Can you work these out from the model? Positions are in its coordinate system, mm. A direction names the side the tool comes from. Coordinates: 2 decimals unless noted, no trailing zeros. Loops run counter-clockwise (first coordinate to the right, second up) from the corner with the lowest first, then second, coordinate; pieces in that order, holes last.
Autodesk Inventor part; units mm, degrees
ref_plane "YZ Plane" through (0, 0, 0) normal (1, 0, 0) x (0, 1, 0)
ref_plane "XZ Plane" through (0, 0, 0) normal (0, 1, 0) x (-1, 0, 0)
ref_plane "XY Plane" through (0, 0, 0) normal (0, 0, 1) x (1, 0, 0)
sketch "Sketch1" plane through (0, 0, 0) normal (0, 0, 1) x (1, 0, 0)
  line L0 (0, 0) -> (18.64, 0)
  line L1 (18.64, 0) -> (18.64, -7)
  line L2 (18.64, -7) -> (0, -7)
  line L3 (0, -7) -> (0, 0)
  circle A0 centre (3.95, -5.19) radius 1.75
  line L4 (9.32, 0) -> (9.32, 1.7268)
  line L5 (9.32, 0) -> (8.32, 0)
  line L6 (8.32, 0) -> (8.32, -6.4)
  line L7 (8.32, -6.4) -> (9.32, -6.4)
  line L8 (9.32, -6.4) -> (9.32, 0)
  circle A1 centre (14.69, -5.19) radius 1.75
  line L9 (10.32, 0) -> (10.32, -6.4)
  line L10 (10.32, -6.4) -> (9.32, -6.4)
  point P0 (8.82, -6.4)
  dimension "d0" = 18.64
  dimension "d1" = 7
  dimension "d2" = 5.19
  dimension "d3" = 3.5
  dimension "d4" = 3.95
  dimension "d5" = 0.6
  dimension "d6" = 1
extrude "Extrusion1" add sketch "Sketch1" along normal blind 1 contours L0 L6 L7 L10 L9 L1 L2 L3
sketch "Sketch2" plane through (0, 0, 1) normal (0, 0, 1) x (1, 0, 0)
  line L0 (0, -7) -> (18.64, -7)
  line L1 (18.64, -7) -> (18.64, 0)
  line L2 (18.64, 0) -> (10.32, 0)
  line L3 (10.32, -6.4) -> (8.32, -6.4)
  line L4 (8.32, -6.4) -> (8.32, 0)
  line L5 (8.32, 0) -> (0, 0)
  line L6 (0, 0) -> (0, -7)
  circle A0 centre (3.95, -5.19) radius 1.75
  circle A1 centre (14.69, -5.19) radius 1.75
  line L7 (8.32, 0) -> (0, 0)
  line L8 (8.32, -6.4) -> (8.32, 0)
  line L9 (0, 0) -> (8.32, 0)
  line L10 (8.32, 0) -> (8.32, -2.5)
  line L11 (8.32, -2.5) -> (0, -2.5)
  line L12 (0, -2.5) -> (0, 0)
  line L13 (9.32, 0) -> (9.32, -6.4)
  line L14 (18.64, -7) -> (18.64, 0)
  line L15 (9.32, 0) -> (18.64, 0)
  line L16 (18.64, 0) -> (18.64, -2.5)
  line L17 (18.64, -2.5) -> (9.32, -2.5)
  line L18 (9.32, -2.5) -> (9.32, 0)
  line L19 (10.32, 0) -> (10.32, -6.4)
  point P0 (0, -2.5)
  point P1 (10.32, -2.5)
  dimension "d9" = 2.5
  dimension "d10" = 2.5
extrude "Extrusion2" add sketch "Sketch2" along normal blind 18 contours L6 L5 L4 L11 | L17 L19 L2 L1
sketch "Sketch3" plane through (8.32, -6.4, 0) normal (1, 0, 0) x (0, 0, -1)
  line L0 (0, 0) -> (0, 6.4)
  line L1 (0, 6.4) -> (-19, 6.4)
  line L2 (-19, 3.9) -> (-19, 6.4)
  line L3 (-1, 3.9) -> (-19, 3.9)
  line L4 (-1, 0) -> (-1, 3.9)
  line L5 (0, 0) -> (-1, 0)
  line L6 (-1, 3.9) -> (-19, 3.9)
  line L7 (-19, 6.4) -> (-9, 6.4)
  line L8 (-9, 6.4) -> (-9, 3.9)
  line L9 (-9, 3.9) -> (-19, 3.9)
  line L10 (-19, 3.9) -> (-19, 6.4)
  point P0 (0, 6.4)
  dimension "d13" = 10
extrude "Extrusion3" add sketch "Sketch3" along normal blind 2 contours L8 L3 L2 L1
sketch "Sketch4" plane through (0, 0, 19) normal (0, 0, 1) x (1, 0, 0)
  line L0 (18.64, 0) -> (10.32, 0)
  line L1 (18.64, 0) -> (0, 0)
  line L2 (0, 0) -> (0, 100)
  line L3 (0, 100) -> (18.64, 100)
  line L4 (18.64, 100) -> (18.64, 0)
  line L5 (10.32, -2.5) -> (10.32, 0)
  line L6 (18.64, 0) -> (0, 0)
  line L7 (0, 0) -> (0, -2.5)
  line L8 (0, -2.5) -> (18.64, -2.5)
  line L9 (18.64, -2.5) -> (18.64, 0)
  dimension "d16" = 100
extrude "Extrusion4" add sketch "Sketch4" along normal blind 2
sketch "Sketch5" plane through (0, 0, 21) normal (0, 0, 1) x (1, 0, 0)
  circle A0 centre (12.82, 93) radius 1.5
  circle A1 centre (5.82, 93) radius 1.5
  line L0 (12.82, 93) -> (5.82, 93)
  line L1 (18.64, 100) -> (0, 100)
  line L2 (9.32, 100) -> (9.32, 93)
  point P0 (0, 0)
  dimension "d19" = 3
  dimension "d20" = 3
  dimension "d21" = 7
  dimension "d22" = 7
extrude "Extrusion5" cut sketch "Sketch5" against normal blind 13.75
sketch "Sketch6" plane through (0, 0, 21) normal (0, 0, 1) x (1, 0, 0)
  line L0 (18.64, 100) -> (0, 100)
  line L1 (9.32, 100) -> (9.32, -19)
  line L2 (9.32, 89) -> (13, 82) construction
  line L3 (13, 82) -> (15, 69) construction
  line L4 (15, 69) -> (15, 40.5) construction
  line L5 (15, 40.5) -> (15, 17) construction
  line L6 (15, 17) -> (12, 4) construction
  line L7 (8.32, 0) -> (10.32, 0)
  line L8 (12, 4) -> (9.32, 0) construction
  spline S0 degree 4 poles (9.32, 89) (13, 82) (15, 69) (15, 40.5) (15, 17) (12, 4) (9.32, 0) knots 1 1 1 1 1 2 3 4 4 4 4 4
  line L9 (9.32, 89) -> (5.64, 82) construction
  line L10 (5.64, 82) -> (3.64, 69) construction
  line L11 (3.64, 69) -> (3.64, 40.5) construction
  line L12 (3.64, 40.5) -> (3.64, 17) construction
  line L13 (3.64, 17) -> (6.64, 4) construction
  line L14 (6.64, 4) -> (9.32, 0) construction
  spline S1 degree 4 poles (9.32, 89) (5.64, 82) (3.64, 69) (3.64, 40.5) (3.64, 17) (6.64, 4) (9.32, 0) knots 1 1 1 1 1 2 3 4 4 4 4 4
  point P0 (0, 0)
extrude "Extrusion6" cut sketch "Sketch6" against normal blind 13.75
fillet "Fillet1" radius 3 2 edges at (0, 100, 20) (18.64, 100, 20)
properties part number "Straight_Distance_Sensor_hold" material "Default New Material"
Item 1: I need wall thicknesses on line 1 along X through (y, z) = (93, 19.4); line 2 along Y through (x, z) = (14, 11.75); line 3 along Z through (x, y) = (15.5, 14). Which ranges of each line are inside material? Lowest first, please.
Results are:
line 1: x = 0 to 4.32, 7.32 to 11.32, 14.32 to 18.64
line 2: y = -2.5 to 0
line 3: z = 19 to 21
Item 2: Suppose I cut it at C-C, the plane y = -5.19. Please give me the cut outline in (x, z), plus the area to 3 significant figures.
Results are:
outline: (0, 0) - (2.2, 0) - (2.2, 1) - (0, 1) - close; (5.7, 0) - (8.32, 0) - (8.32, 1) - (5.7, 1) - close; (10.32, 0) - (12.94, 0) - (12.94, 1) - (10.32, 1) - close; (16.44, 0) - (18.64, 0) - (18.64, 1) - (16.44, 1) - close
area: 9.64 mm2
Item 3: Suppose I cut it at A-A, the plane y = 93. Please give me the cut outline in (x, z).
Results are:
outline: (0, 19) - (4.32, 19) - (4.32, 21) - (0, 21) - close; (7.32, 19) - (11.32, 19) - (11.32, 21) - (7.32, 21) - close; (14.32, 19) - (18.64, 19) - (18.64, 21) - (14.32, 21) - close
Item 4: I'm going to push flat-ended pins straight in: P1, Ø5, axis at y = -3, z = 6, coming from the -X side; P2, Ø1, axis at x = 12.5, z = 13.5, coming from the +Y side; P3, Ø5.5, axis at x = 13, y = 74.5, coming from the -Z side; P4, Ø4, axis at x = 3.5, z = 13, coming from the -Y side. Where does each tip first touch, or does it pass through?
Results are:
P1: stops at x = 0
P2: stops at y = 0
P3: stops at z = 19
P4: stops at y = -2.5
Item 5: We'd pull the mould along Y, two halves only. Please class faces 1 (the face through (17.78, 99.1, 20.01)), 2 (the face through (7, -5, 1)), 3 (the face through (12.625, 94.487, 20.014)): +Y half, -Y half, draft (parallel to the pull), parting line (faces both ways), or undercut.
Results are:
face 1: +Y half
face 2: draft
face 3: undercut
Item 6: Suppose I cut it at B-B, the plane z = 5.5. Please give me the cut outline in (x, y).
Results are:
outline: (0, -2.5) - (8.32, -2.5) - (8.32, 0) - (0, 0) - close; (10.32, -2.5) - (18.64, -2.5) - (18.64, 0) - (10.32, 0) - close
Item 7: On a 3-axis mill with a long thin cutter (end or side, diameter ignored), from which of +Z, -Z, +X, -X, +Y, -Y can I reach the whole of each face in a straight line? I mean faces 4 (the face through (10.32, -2, 4)), 5 (the face through (9, -1, 9)), 6 (the face through (16.3, -4.5, 0.5)), 7 (the face through (9, -2.5, 11)), 8 (the face through (3, 51, 19)). Say none if no direction works.
Results are:
face 4: -Z, +Y
face 5: -Z, +Y, -Y
face 6: +Z, -Z
face 7: +Z, +X, -X, -Y
face 8: -Z, +X, -X, +Y
Item 8: Suppose I cut it at D-D, the plane z = 11. Please give me the cut outline in (x, y).
Results are:
outline: (0, -2.5) - (18.64, -2.5) - (18.64, 0) - (0, 0) - close
